Check sheet for the drawn part. Datum: minimum x, y, z corner. Units: mm. A direction names the side the tool comes from. Coordinates: 2 decimals unless noted, no trailing zeros. Loops run counter-clockwise (first coordinate to the right, second up) from the corner with the lowest first, then second, coordinate; pieces in that order, holes last.
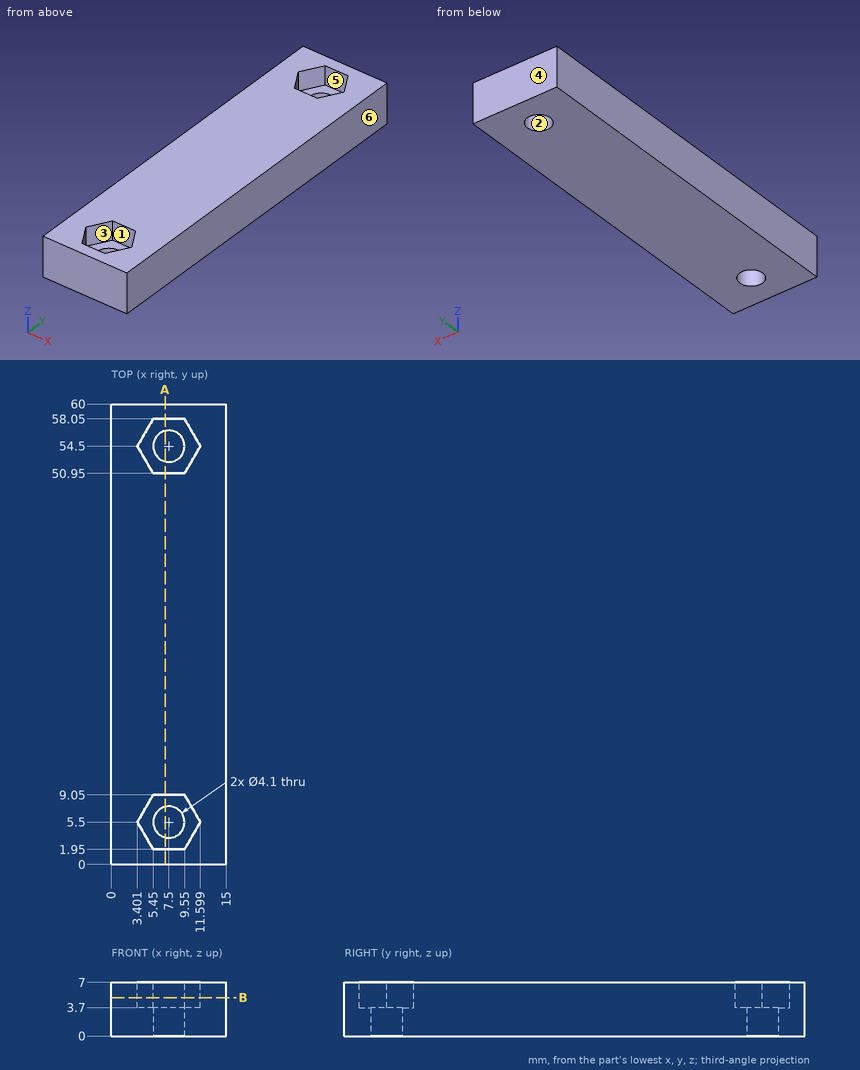
(1) Sectioned sample at B-B on z = 5. Record the cut outline in (x, y), and give its area (3 significant figures).
Findings:
outline: (0, 0) - (15, 0) - (15, 60) - (0, 60) - close; hole (3.4, 5.5) - (5.45, 1.95) - (9.55, 1.95) - (11.6, 5.5) - (9.55, 9.05) - (5.45, 9.05) - close; hole (3.4, 54.5) - (5.45, 50.95) - (9.55, 50.95) - (11.6, 54.5) - (9.55, 58.05) - (5.45, 58.05) - close
area: 813 mm2
(2) Sectioned sample at A-A on x = 7. Record the cut outline in (y, z).
Findings:
outline: (0, 0) - (3.51, 0) - (3.51, 3.7) - (1.95, 3.7) - (1.95, 7) - (0, 7) - close; (7.49, 0) - (52.51, 0) - (52.51, 3.7) - (50.95, 3.7) - (50.95, 7) - (9.05, 7) - (9.05, 3.7) - (7.49, 3.7) - close; (56.49, 0) - (60, 0) - (60, 7) - (58.05, 7) - (58.05, 3.7) - (56.49, 3.7) - close
(3) Gauge pin test, flat ends, axial feed: pin 1 Ø6.5 at (x, y) = (7.5, 5.5) entering from +Z; pin 2 Ø3.5 at (x, y) = (7.5, 54.5) entering from +Z. Record the tip position at first contact, or that the pin passes through.
Findings:
pin 1: stops at z = 3.7
pin 2: passes through
(4) Scan lines: L1, parallel to Y at x = 7.5, z = 2.45; L2, parallel to Y at x = 6.75, z = 5.5; L3, parallel to X at y = 4.5, z = 4. Record each from-to range of solid material in increasing order.
Findings:
L1: y = 0 to 3.45, 7.55 to 52.45, 56.55 to 60
L2: y = 0 to 1.95, 9.05 to 50.95, 58.05 to 60
L3: x = 0 to 3.98, 11.02 to 15
(5) Draft check along Y on the marked faces 3, 4, 5 and 6. Enter one of: +Y half, -Y half, draft (parallel to the pull), parting line (faces both ways), or undercut.
Findings:
face 3: undercut
face 4: +Y half
face 5: undercut
face 6: draft
(6) Access from +Z, -Z, +X, -X, +Y, -Y to the whole of each face (thin tool, end or side, straight path). Record for the marked faces 1 and 2.
Findings:
face 1: +Z
face 2: +Z, -Z
